```python
from build123d import *

# Parameters (mm, degrees)
SKETCH_1_W           = 176
SKETCH_1_H           = 120
EXTRUDE_1_DEPTH      = 10
SKETCH_2_W           = 171
SKETCH_2_H           = 112
CUT_EXTRUDE_1_DEPTH  = 1.8
SKETCH_3_W           = 171
SKETCH_3_H           = 112
CUT_EXTRUDE_2_DEPTH  = 1.8
SKETCH_5_W           = 173.4
SKETCH_5_H           = 116
CUT_EXTRUDE_3_DEPTH  = 0.5
SKETCH_6_W           = 173.4
SKETCH_6_H           = 116
CUT_EXTRUDE_4_DEPTH  = 0.5
SKETCH_7_W           = 32.5
SKETCH_7_H           = 56
CUT_EXTRUDE_5_DEPTH  = 107.823405675
SKETCH_8_W           = 12.5
SKETCH_8_H           = 44
CUT_EXTRUDE_6_DEPTH  = 0.5
SKETCH_9_W           = 12.5
SKETCH_9_H           = 44
CUT_EXTRUDE_7_DEPTH  = 0.5
SKETCH_10_W          = 25
SKETCH_10_H          = 12
CUT_EXTRUDE_8_DEPTH  = 0.8
CUT_EXTRUDE_10_DEPTH = 6
FILLET_1_R           = 4
FILLET_2_R           = 4
SKETCH_18_W          = 1.5
SKETCH_18_H          = 3
EXTRUDE_3_DEPTH      = 2.5
SKETCH_20_W          = 1.5
SKETCH_20_H          = 3
EXTRUDE_4_DEPTH      = 2.5
SKETCH_21_W          = 12.5
SKETCH_21_H          = 16
CUT_EXTRUDE_12_DEPTH = 107.786188245
SKETCH_22_W          = 25
SKETCH_22_H          = 10
CUT_EXTRUDE_13_DEPTH = 4.5
SKETCH_23_W          = 25
SKETCH_23_H          = 2
EXTRUDE_5_DEPTH      = 0.8
FILLET_15_R          = 0.5
EXTRUDE_START        = 2.5
EXTRUDE_6_DEPTH      = 2.5
SKETCH_25_W          = 12.5
SKETCH_25_H          = 10.082968054
CUT_EXTRUDE_14_DEPTH = 1.4
SKETCH_26_W          = 12.5
SKETCH_26_H          = 10.082968054
CUT_EXTRUDE_15_DEPTH = 1.4
FILLET_16_R          = 1
FILLET_17_R          = 1
FILLET_18_R          = 1
FILLET_19_R          = 1
FILLET_21_R          = 2
FILLET_22_R          = 2
SKETCH_28_R          = 2.75
CUT_EXTRUDE_16_DEPTH = 5.5
FILLET_23_R          = 0.5


with BuildPart() as part:
    # 草图1 → 凸台-拉伸1 (new body)
    with BuildSketch(Plane.XY):
        Rectangle(SKETCH_1_W, SKETCH_1_H)
    extrude(amount=EXTRUDE_1_DEPTH)

    # 草图2 → 切除-拉伸1 (cut)
    with BuildSketch(Plane.XY.offset(10)):
        Rectangle(SKETCH_2_W, SKETCH_2_H)
    extrude(amount=-CUT_EXTRUDE_1_DEPTH, mode=Mode.SUBTRACT)

    # 草图3 → 切除-拉伸2 (cut)
    with BuildSketch(Plane(origin=(0, 0, 0), x_dir=(-1, 0, 0), z_dir=(0, 0, -1))):
        Rectangle(SKETCH_3_W, SKETCH_3_H)
    extrude(amount=-CUT_EXTRUDE_2_DEPTH, mode=Mode.SUBTRACT)

    # 草图5 → 切除-拉伸3 (cut)
    with BuildSketch(Plane(origin=(0, 0, 0), x_dir=(-1, 0, 0), z_dir=(0, 0, -1))):
        Rectangle(SKETCH_5_W, SKETCH_5_H)
    extrude(amount=-CUT_EXTRUDE_3_DEPTH, mode=Mode.SUBTRACT)

    # 草图6 → 切除-拉伸4 (cut)
    with BuildSketch(Plane.XY.offset(10)):
        Rectangle(SKETCH_6_W, SKETCH_6_H)
    extrude(amount=-CUT_EXTRUDE_4_DEPTH, mode=Mode.SUBTRACT)

    # 草图7 → 切除-拉伸5 (cut, through all)
    with BuildSketch(Plane(origin=(0, 0, 1.8), x_dir=(-1, 0, 0), z_dir=(0, 0, -1))):
        with Locations((0, 16)):
            Rectangle(SKETCH_7_W, SKETCH_7_H)
    extrude(amount=-CUT_EXTRUDE_5_DEPTH, mode=Mode.SUBTRACT)

    # 草图8 → 切除-拉伸6 (cut)
    with BuildSketch(Plane(origin=(0, 0, 1.8), x_dir=(-1, 0, 0), z_dir=(0, 0, -1))):
        with Locations((0, -34)):
            Rectangle(SKETCH_8_W, SKETCH_8_H)
    extrude(amount=-CUT_EXTRUDE_6_DEPTH, mode=Mode.SUBTRACT)

    # 草图9 → 切除-拉伸7 (cut)
    with BuildSketch(Plane.XY.offset(8.2)):
        with Locations((0, -34)):
            Rectangle(SKETCH_9_W, SKETCH_9_H)
    extrude(amount=-CUT_EXTRUDE_7_DEPTH, mode=Mode.SUBTRACT)

    # 草图10 → 切除-拉伸8 (cut)
    with BuildSketch(Plane.XY.offset(8.2)):
        with Locations((0, 50)):
            Rectangle(SKETCH_10_W, SKETCH_10_H)
    extrude(amount=-CUT_EXTRUDE_8_DEPTH, mode=Mode.SUBTRACT)

    # 草图13 → 切除-拉伸10 (cut)
    with BuildSketch(Plane(origin=(0, 60, 0), x_dir=(1, 0, 0), z_dir=(0, 1, 0))):
        with BuildLine():
            Line((-13.75, -2.75), (13.75, -2.75))
            ThreePointArc((13.75, -2.75), (16, -5), (13.75, -7.25))
            Line((13.75, -7.25), (-13.75, -7.25))
            ThreePointArc((-13.75, -7.25), (-16, -5), (-13.75, -2.75))
        make_face()
    extrude(amount=-CUT_EXTRUDE_10_DEPTH, mode=Mode.SUBTRACT)

    # 圆角1
    fillet_1_edges = [part.edges().sort_by_distance(p)[0] for p in [
        (-88, 60, 5),
    ]]
    fillet(fillet_1_edges, radius=FILLET_1_R)

    # 圆角2
    fillet_2_edges = [part.edges().sort_by_distance(p)[0] for p in [
        (88, 60, 5),
    ]]
    fillet(fillet_2_edges, radius=FILLET_2_R)

    # 草图18 → 凸台-拉伸3 (add)
    with BuildSketch(Plane(origin=(-16.25, 0, 0), x_dir=(0, 0, -1), z_dir=(1, 0, 0))):
        with Locations((-2.55, -10.5)):
            Rectangle(SKETCH_18_W, SKETCH_18_H)
        with Locations((-7.45, -10.5)):
            Rectangle(SKETCH_18_W, SKETCH_18_H)
    extrude(amount=EXTRUDE_3_DEPTH)

    # 草图20 → 凸台-拉伸4 (add)
    with BuildSketch(Plane.ZY.offset(-16.25)):
        with Locations((7.45, -10.5)):
            Rectangle(SKETCH_20_W, SKETCH_20_H)
        with Locations((2.55, -10.5)):
            Rectangle(SKETCH_20_W, SKETCH_20_H)
    extrude(amount=EXTRUDE_4_DEPTH)

    # 草图21 → 切除-拉伸12 (cut, through all)
    with BuildSketch(Plane(origin=(0, 0, 2.3), x_dir=(-1, 0, 0), z_dir=(0, 0, -1))):
        with Locations((0, -30.082968054)):
            Rectangle(SKETCH_21_W, SKETCH_21_H)
    extrude(amount=-CUT_EXTRUDE_12_DEPTH, mode=Mode.SUBTRACT)

    # 草图22 → 切除-拉伸13 (cut)
    with BuildSketch(Plane.XY.offset(7.4)):
        with Locations((0, 49)):
            Rectangle(SKETCH_22_W, SKETCH_22_H)
    extrude(amount=-CUT_EXTRUDE_13_DEPTH, mode=Mode.SUBTRACT)

    # 草图23 → 凸台-拉伸5 (add)
    with BuildSketch(Plane.XY.offset(7.4)):
        with Locations((0, 55)):
            Rectangle(SKETCH_23_W, SKETCH_23_H)
    extrude(amount=EXTRUDE_5_DEPTH)

    # 圆角15
    fillet_15_edges = [part.edges().sort_by_distance(p)[0] for p in [
        (0, 54, 7.25),
    ]]
    fillet(fillet_15_edges, radius=FILLET_15_R)

    # 草图24 → 凸台-拉伸6 (add)
    with BuildSketch(Plane(origin=(0, 54, 0), x_dir=(1, 0, 0), z_dir=(0, 1, 0)).offset(EXTRUDE_START)):
        with BuildLine():
            Line((-13.75, -2.75), (-13.75, -7.25))
            ThreePointArc((-13.75, -7.25), (-16, -5), (-13.75, -2.75))
        make_face()
        with BuildLine():
            Line((13.75, -2.75), (13.75, -7.25))
            ThreePointArc((13.75, -7.25), (16, -5), (13.75, -2.75))
        make_face()
    extrude(amount=-EXTRUDE_6_DEPTH)

    # 草图25 → 切除-拉伸14 (cut)
    with BuildSketch(Plane.XY.offset(7.7)):
        with Locations((0, -17.041484027)):
            Rectangle(SKETCH_25_W, SKETCH_25_H)
    extrude(amount=-CUT_EXTRUDE_14_DEPTH, mode=Mode.SUBTRACT)

    # 草图26 → 切除-拉伸15 (cut)
    with BuildSketch(Plane(origin=(0, 0, 2.3), x_dir=(-1, 0, 0), z_dir=(0, 0, -1))):
        with Locations((0, -17.041484027)):
            Rectangle(SKETCH_26_W, SKETCH_26_H)
    extrude(amount=-CUT_EXTRUDE_15_DEPTH, mode=Mode.SUBTRACT)

    # 圆角16
    fillet_16_edges = [part.edges().sort_by_distance(p)[0] for p in [
        (0, -22.082968054, 3.7),
    ]]
    fillet(fillet_16_edges, radius=FILLET_16_R)

    # 圆角17
    fillet_17_edges = [part.edges().sort_by_distance(p)[0] for p in [
        (0, -12, 3.7),
    ]]
    fillet(fillet_17_edges, radius=FILLET_17_R)

    # 圆角18
    fillet_18_edges = [part.edges().sort_by_distance(p)[0] for p in [
        (0, -12, 6.3),
    ]]
    fillet(fillet_18_edges, radius=FILLET_18_R)

    # 圆角19
    fillet_19_edges = [part.edges().sort_by_distance(p)[0] for p in [
        (0, -22.082968054, 6.3),
    ]]
    fillet(fillet_19_edges, radius=FILLET_19_R)

    # 圆角21
    fillet_21_edges = [part.edges().sort_by_distance(p)[0] for p in [
        (0, -38.082968054, 7.7),
    ]]
    fillet(fillet_21_edges, radius=FILLET_21_R)

    # 圆角22
    fillet_22_edges = [part.edges().sort_by_distance(p)[0] for p in [
        (0, -38.082968054, 2.3),
    ]]
    fillet(fillet_22_edges, radius=FILLET_22_R)

    # 草图28 → 切除-拉伸16 (cut)
    with BuildSketch(Plane(origin=(0, -60, 0), x_dir=(-1, 0, 0), z_dir=(0, -1, 0))):
        with Locations(Location((-72, -5, 0), (0, 0, 180))):
            Circle(SKETCH_28_R)
        with Locations(Location((-38, -5, 0), (0, 0, 180))):
            Circle(SKETCH_28_R)
        with Locations(Location((38, -5, 0), (0, 0, 180))):
            Circle(SKETCH_28_R)
        with Locations(Location((72, -5, 0), (0, 0, 180))):
            Circle(SKETCH_28_R)
    extrude(amount=-CUT_EXTRUDE_16_DEPTH, mode=Mode.SUBTRACT)

    # 圆角23
    fillet_23_edges = [part.edges().sort_by_distance(p)[0] for p in [
        (0, 44, 2.9),
    ]]
    fillet(fillet_23_edges, radius=FILLET_23_R)


solid = part.part
```
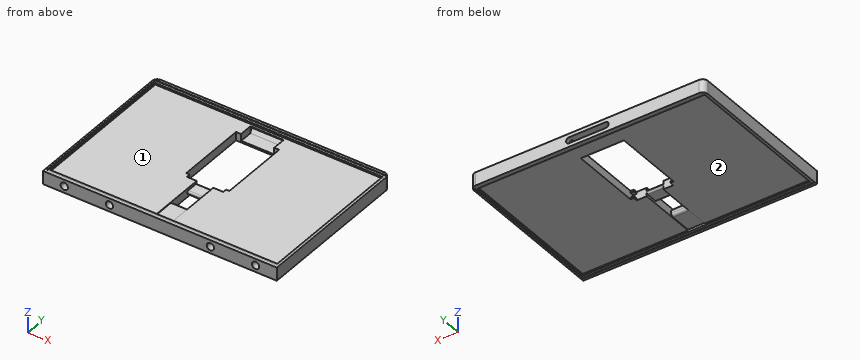
Geometry: final body of the model. Coordinates: model frame, mm. Face numbers are marked on the shaded views. A direction names the side the tool comes from. Coordinates: 2 decimals unless noted, no trailing zeros. Order: outer loops, then holes, each group sorted by start corner. A loop starts at its lowest first (then second) coordinate and runs counter-clockwise, first axis right, second up. Notation, with made-up numbers: (70.25, -1) - (83.25, -1) arc R37 ccw to (83.25, 37) - close; hole circle Ø9 at (-28.75, 53). An arc over 180 degrees is marked (long way). Write each question's results on one line, items separated by ' | '.
(1) Section query A-A, the plane x = 24. Return the cut outline in (y, z), plus the area to 3 significant figures.
Values found:
outline: (-60, 0) - (-58, 0) - (-58, 0.5) - (-56, 0.5) - (-56, 1.8) - (56, 1.8) - (56, 0.5) - (58, 0.5) - (58, 0) - (60, 0) - (60, 10) - (58, 10) - (58, 9.5) - (56, 9.5) - (56, 8.2) - (-56, 8.2) - (-56, 9.5) - (-58, 9.5) - (-58, 10) - (-60, 10) - close | area: 793 mm²
(2) Section query C-C, the plane x = -38. Return the cut outline in (y, z).
Values found:
outline: (-60, 0) - (-58, 0) - (-58, 0.5) - (-56, 0.5) - (-56, 1.8) - (56, 1.8) - (56, 0.5) - (58, 0.5) - (58, 0) - (60, 0) - (60, 10) - (58, 10) - (58, 9.5) - (56, 9.5) - (56, 8.2) - (-56, 8.2) - (-56, 9.5) - (-58, 9.5) - (-58, 10) - (-60, 10) - (-60, 7.75) - (-54.5, 7.75) - (-54.5, 2.25) - (-60, 2.25) - close
(3) Section query B-B, the plane y = -47. Return the cut outline in (x, z), plus the area to 3 significant figures.
Values found:
outline: (-88, 0) - (-86.7, 0) - (-86.7, 0.5) - (-85.5, 0.5) - (-85.5, 1.8) - (-6.25, 1.8) - (-6.25, 2.3) - (6.25, 2.3) - (6.25, 1.8) - (85.5, 1.8) - (85.5, 0.5) - (86.7, 0.5) - (86.7, 0) - (88, 0) - (88, 10) - (86.7, 10) - (86.7, 9.5) - (85.5, 9.5) - (85.5, 8.2) - (6.25, 8.2) - (6.25, 7.7) - (-6.25, 7.7) - (-6.25, 8.2) - (-85.5, 8.2) - (-85.5, 9.5) - (-86.7, 9.5) - (-86.7, 10) - (-88, 10) - close | area: 1,130 mm²
(4) First-contact query: pin 1 Ø5 at (x, z) = (11.5, 6.5) entering from +Y; pin 2 Ø5 at (x, y) = (44.5, -24.5) entering from -Z; pin 3 Ø5 at (x, y) = (-43, -7.5) entering from +Z; pin 4 Ø1.1 at (x, z) = (-2.5, 5) entering from +Y. Flat tips, straight axial feed; report the tip coordinate or a pass-through.
Values found:
pin 1: stops at y = 60 | pin 2: stops at z = 1.8 | pin 3: stops at z = 8.2 | pin 4: stops at y = -12
(5) Set-up query: the marked faces 1 and 2. Return all of +Z, -Z, +X, -X, +Y, -Y with unobstructed straight access to the full face (end or side cutting, diameter ignored); none if empty.
Values found:
face 1: +Z | face 2: -Z
(6) Line query: line 1 (Z direction, x = -72, y = -55); line 2 (X direction, y = -28.5, z = 9.75); line 3 (X direction, y = -9, z = 5). Output: solid intervals per line, ascending. Write a range as [from, to].
Values found:
line 1: z = [1.8, 2.25], [7.75, 8.2] | line 2: x = [-88, -86.7], [86.7, 88] | line 3: x = [-88, -16.25], [16.25, 88]
